Autodesk Inventor part; units mm, degrees
ref_plane "YZ Plane" through (0, 0, 0) normal (1, 0, 0) x (0, 1, 0)
ref_plane "XZ Plane" through (0, 0, 0) normal (0, 1, 0) x (-1, 0, 0)
ref_plane "XY Plane" through (0, 0, 0) normal (0, 0, 1) x (1, 0, 0)
sketch "Sketch1" plane through (0, 0, 0) normal (1, 0, 0) x (0, 1, 0)
  line L0 (0, 0) -> (500, 0)
  line L1 (500, 0) -> (500, -300)
  line L2 (500, -300) -> (0, -300)
  line L3 (0, -300) -> (0, 0)
  dimension "d0" = 300
  dimension "d1" = 500
extrude "Extrusion1" add sketch "Sketch1" along normal blind 5
sketch "Sketch2" plane through (0, 0, -300) normal (0, 0, -1) x (-1, 0, 0)
  line L0 (0, 0) -> (-100, 0)
  line L1 (-100, 0) -> (-100, 500)
  line L2 (-100, 500) -> (0, 500)
  line L3 (0, 500) -> (0, 0)
  point P0 (-50, 0)
  dimension "d4" = 100
  dimension "d5" = 500
extrude "Extrusion2" add sketch "Sketch2" along normal blind 5
sketch "Sketch3" plane through (0, 0, -305) normal (0, 0, -1) x (-1, 0, 0)
  circle A0 centre (-88, 400) radius 5
  line L0 (-100, 500) -> (-100, 0)
  line L1 (0, 500) -> (-100, 500)
  point P0 (0, 0)
  dimension "d8" = 10
  dimension "d9" = 12
  dimension "d10" = 100
extrude "Extrusion3" cut sketch "Sketch3" against normal blind 5
properties part number "door"
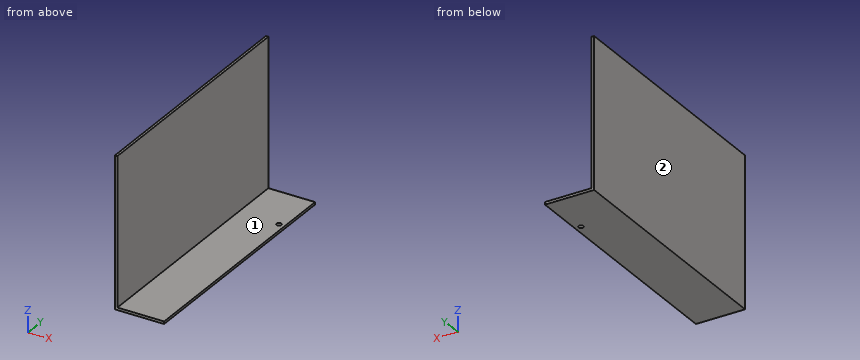
Read the model definition and answer for the solid it produces. Units are mm, in the model's axes. Face numbers are marked on the shaded views. A direction names the side the tool comes from. Round coordinates to 2 decimals unless told otherwise and drop trailing zeros. Write each loop counter-clockwise with the first axis right and the second up, starting at its lowest first coordinate (ties: lowest second). Pieces come first, ordered by that corner, then holes. Notation, with made-up numbers: M -37.75,7 L -6.75,7 A19 cw -6.75,11 Z; hole C -4.5,-37.75 d6. An arc over 180 degrees is marked long. One line per item, written item: value.
Q1. Which of the six approach directions +Z, -Z, +X, -X, +Y, -Y give full straight-line access (tool end or side, diameter ignored) to the marked faces 1 and 2?
Data:
face 1: +Z, +X, +Y, -Y
face 2: +Z, -Z, -X, +Y, -Y
Q2. Find section A-A on x = 88. Write down the section's boundary in (y, z).
Data:
outline: M 0,-305 L 395,-305 L 395,-300 L 0,-300 Z; M 405,-305 L 500,-305 L 500,-300 L 405,-300 Z
Q3. Find section C-C on y = 156. Write down the section's boundary in (x, z), plus the area to 3 significant figures.
Data:
outline: M 0,-305 L 100,-305 L 100,-300 L 5,-300 L 5,0 L 0,0 Z
area: 2,000 mm2
Q4. Find section B-B on y = 400. Write down the section's boundary in (x, z).
Data:
outline: M 0,-305 L 83,-305 L 83,-300 L 5,-300 L 5,0 L 0,0 Z; M 93,-305 L 100,-305 L 100,-300 L 93,-300 Z
Q5. Find section D-D on x = 24. Write down the section's boundary in (y, z).
Data:
outline: M 0,-305 L 500,-305 L 500,-300 L 0,-300 Z
Q6. Flat-ended cylindrical pins translate along their axes: pin 1 Ø1.5 at (y, z) = (335, -256.5) entering from +X; pin 2 Ø8 at (x, y) = (33, 406) entering from +Z; pin 3 Ø8 at (x, y) = (88, 400) entering from -Z. Find the tip coordinate at first contact, or state that the pin passes through.
Data:
pin 1: x = 5
pin 2: z = -300
pin 3: through
Q7. Straight lines are drawn through the part: line 1 (Y direction, x = 88, z = -301.95); line 2 (X direction, y = 400, z = -301); line 3 (Z direction, x = 54, y = 167). For each, find the intervals that lie inside material, in ascending order. Write a range as [from, to].
Data:
line 1: [0, 395], [405, 500]
line 2: [0, 83], [93, 100]
line 3: [-305, -300]
